Here's how the part is built. I have some questions about the finished solid (model axes, mm). Give positions to 0.01 mm unless a question says otherwise; leave off trailing zeros. Write each loop counter-clockwise with the first axis right and the second up, starting at its lowest first coordinate (ties: lowest second). Pieces come first, ordered by that corner, then holes. Notation, with made-up numbers: (24, 50.5) - (39, 50.5) arc R15 cw to (39, 70.5) - close; hole circle Ø5 at (-3.75, -36). An arc over 180 degrees is marked (long way). One line per item, written item: value. Start each with the question number.
1) Imagine slicing it at D-D on y = -14.75. Write out the boundary of the cut face in (x, z), plus the area to 3 significant figures.
2) Imagine slicing it at B-B on x = 25. Write out the boundary of the cut face in (y, z).
3) Imagine slicing it at C-C on z = -50. Write out the boundary of the cut face in (x, y).
4) We'd pull the mould along Z, two halves only. Please class faces 1 (the cylindrical face through (-2.288, -12.522, 85.798)), 2 (the flat face through (-1, -13, -76.291)), 3 (the flat face through (-49.308, -13, 6)), 4 (the flat face through (-1, -13, 91.027)): +Z half, -Z half, draft (parallel to the pull), parting line (faces both ways), or undercut.
5) Please list where these lines run through material, in increasing order: L1, parallel to Z at x = 0, y = -15.75; L2, parallel to Z at x = -3, y = -1; L3, parallel to Z at x = -26.5, y = -10. Write a range as [from, to].
6) Imagine slicing it at A-A on x = 0. Write out the boundary of the cut face in (y, z), plus the area to 3 significant figures.
from build123d import *

# Parameters (mm, degrees)
F0_W     = 98.944682
F0_H     = 167.318415
F0_R     = 17.573737
F1_DEPTH = 25.4


with BuildPart() as f1:
    # F0 (on Front) → F1 (new body)
    with BuildSketch(Plane.XZ):
        with Locations((0.164358, 7.368268)):
            Rectangle(F0_W, F0_H)
        with BuildLine():
            ThreePointArc((-6.892271, -37.47141), (-24.382519, 29.276318), (38.1, 0))
            ThreePointArc((38.1, 0), (29.276318, -24.382519), (6.892271, -37.47141))
            ThreePointArc((6.892271, -37.47141), (14.662183, -43.949239), (17.573737, -53.637203))
            ThreePointArc((17.573737, -53.637203), (-9.687964, -68.299385), (-6.892271, -37.47141))
        make_face(mode=Mode.SUBTRACT)
        with Locations((0, 68.373737)):
            Circle(F0_R, mode=Mode.SUBTRACT)
    extrude(amount=F1_DEPTH)


solid = f1.part
Numbers:
1. outline: (-49.31, -76.29) - (49.64, -76.29) - (49.64, 91.03) - (-49.31, 91.03) - close; hole circle Ø35.15 at (0, 68.37); hole (-6.89, -37.47) arc R17.57 ccw (long way) to (17.57, -53.64) arc R17.57 ccw to (6.89, -37.47) arc R38.1 ccw to (38.1, 0) arc R38.1 ccw (long way) to start
1. area: 10,100 mm^2
2. outline: (-25.4, -76.29) - (0, -76.29) - (0, -28.75) - (-25.4, -28.75) - close; (-25.4, 28.75) - (0, 28.75) - (0, 91.03) - (-25.4, 91.03) - close
3. outline: (-49.31, -25.4) - (-17.19, -25.4) - (-17.19, 0) - (-49.31, 0) - close; (17.19, -25.4) - (49.64, -25.4) - (49.64, 0) - (17.19, 0) - close
4. face 1: undercut
4. face 2: -Z half
4. face 3: draft
4. face 4: +Z half
5. L1: [-76.29, -71.21], [38.1, 50.8], [85.95, 91.03]
5. L2: [-76.29, -70.95], [37.98, 51.06], [85.69, 91.03]
5. L3: [-76.29, -27.37], [27.37, 91.03]
6. outline: (-25.4, -76.29) - (0, -76.29) - (0, -71.21) - (-25.4, -71.21) - close; (-25.4, 38.1) - (0, 38.1) - (0, 50.8) - (-25.4, 50.8) - close; (-25.4, 85.95) - (0, 85.95) - (0, 91.03) - (-25.4, 91.03) - close
6. area: 581 mm^2
